Autodesk Inventor part; units mm, degrees
ref_plane "YZ Plane" through (0, 0, 0) normal (1, 0, 0) x (0, 1, 0)
ref_plane "XZ Plane" through (0, 0, 0) normal (0, 1, 0) x (-1, 0, 0)
ref_plane "XY Plane" through (0, 0, 0) normal (0, 0, 1) x (1, 0, 0)
ref_plane "Work Plane1" through (0, 0, 152.1968) normal (0, 0, 1) x (1, 0, 0)
sketch "Sketch2" plane through (0, 0, 152.1968) normal (0, 0, 1) x (1, 0, 0)
  line L0 (0, 0) -> (152.1206, 0)
  line L1 (152.1206, 0) -> (152.1206, 6.35)
  line L2 (152.1206, 6.35) -> (0, 6.35)
  line L3 (0, 6.35) -> (0, 0)
  dimension "d20" = 152.1206
  dimension "d21" = 6.35
extrude "Extrusion2" add sketch "Sketch2" along normal blind 69.85
sketch "Sketch4" plane through (0, 6.35, 152.1968) normal (0, 1, 0) x (1, 0, 0)
  circle A0 centre (19.05, -3.175) radius 1.5875
  circle A1 centre (133.0706, -3.175) radius 1.5875
  circle A2 centre (133.0706, -66.675) radius 1.5875
  circle A3 centre (19.05, -66.675) radius 1.5875
  line L0 (0, 0) -> (0, -69.85)
  line L1 (152.1206, 0) -> (0, 0)
  line L2 (152.1206, 0) -> (152.1206, -69.85)
  line L3 (152.1206, -69.85) -> (0, -69.85)
  point P0 (0, 152.1968)
  dimension "d22" = 3.175
  dimension "d23" = 19.05
  dimension "d24" = 3.175
  dimension "d25" = 19.05
  dimension "d26" = 3.175
extrude "Extrusion4" cut sketch "Sketch4" against normal blind 152.1968 contours A0 | A1 | A2 | A3
properties part number "Base"
Geometry: final body of the model. Coordinates: model frame, mm. Round coordinates to 2 decimals unless told otherwise and drop trailing zeros. Order: outer loops, then holes, each group sorted by start corner. A loop starts at its lowest first (then second) coordinate and runs counter-clockwise, first axis right, second up. Notation, with made-up numbers: (40.5, 81.5) -> (51.5, 81.5) arc R25 ccw to (51.5, 101.5) -> close; hole circle Ø7 at (-1, 52.5). An arc over 180 degrees is marked (long way). Put each result on its own line as item: value. Start each with the question number.
Q1. Line query: probe 1 along Z at (x, y) = (19, 5.5); probe 2 along X at (y, z) = (2, 218.5). Output: solid intervals per line, ascending.
Q2. First-contact query: pin 1 (1.9 mm diameter, centred on x = 133.07, z = 155.37, fed in from +Y). Flat tip, straight axial feed; report the tip coordinate or a pass-through.
Q3. Section A-A on x = 19.05. Return the cut outline in (y, z).
Q4. Pull-direction query (Z, two-part tool) for faces 1 (the flat face through (0, 3, 187)), 2 (the cylindrical face through (18.84, 3.22, 217.3)), 3 (the flat face through (75, 3, 222.047)); classes: +Z half, -Z half, draft (parallel to the pull), parting line (faces both ways), or undercut.
Ans:
1. probe 1: z = 152.2 to 153.79, 156.96 to 217.29, 220.46 to 222.05
1. probe 2: x = 0 to 17.51, 20.59 to 131.53, 134.61 to 152.12
2. pin 1: passes through
3. outline: (0, 152.2) -> (6.35, 152.2) -> (6.35, 153.78) -> (0, 153.78) -> close; (0, 156.96) -> (6.35, 156.96) -> (6.35, 217.28) -> (0, 217.28) -> close; (0, 220.46) -> (6.35, 220.46) -> (6.35, 222.05) -> (0, 222.05) -> close
4. face 1: draft
4. face 2: undercut
4. face 3: +Z half
